from build123d import *

# Parameters (mm, degrees)
SKETCH1_R               = 20
BOSS_EXTRUDE1_DEPTH     = 142.5
SKETCH2_R               = 24
BOSS_EXTRUDE2_DEPTH     = 15
SKETCH3_R               = 20
BOSS_EXTRUDE3_DEPTH     = 40
SKETCH5_R               = 15
BOSS_EXTRUDE4_DEPTH     = 45
CUT_EXTRUDE1_DEPTH      = 245.863737617
CUT_EXTRUDE1_DEPTH_BACK = 245.863737617
SKETCH4_R               = 11.5
SKETCH7_W               = 2
SKETCH7_H               = 1.5
SKETCH10_W              = 2.5
SKETCH10_H              = 50.5


with BuildPart() as part:
    # Sketch1 → Boss-Extrude1 (new body)
    with BuildSketch(Plane(origin=(0, 0, 0), x_dir=(1, 0, 0), z_dir=(0, 1, 0))):
        with Locations(Location((0, 0, 0), (0, 0, 270))):
            Circle(SKETCH1_R)
    extrude(amount=BOSS_EXTRUDE1_DEPTH)

    # Sketch2 → Boss-Extrude2 (add)
    with BuildSketch(Plane(origin=(0, 142.5, 0), x_dir=(1, 0, 0), z_dir=(0, 1, 0))):
        with Locations(Location((0, 0, 0), (0, 0, 270))):
            Circle(SKETCH2_R)
    extrude(amount=BOSS_EXTRUDE2_DEPTH)

    # Sketch3 → Boss-Extrude3 (add)
    with BuildSketch(Plane(origin=(0, 157.5, 0), x_dir=(1, 0, 0), z_dir=(0, 1, 0))):
        with Locations(Location((-0.463755605, 0, 0), (0, 0, 270))):
            Circle(SKETCH3_R)
    extrude(amount=BOSS_EXTRUDE3_DEPTH)

    # Sketch5 → Boss-Extrude4 (add)
    with BuildSketch(Plane.XZ):
        with Locations(Location((0, 0, 0), (0, 0, 90))):
            Circle(SKETCH5_R)
    extrude(amount=BOSS_EXTRUDE4_DEPTH)

    # Sketch4 → Cut-Extrude1 (cut, two sides: drawn at the far end of the back side and taken through both)
    with BuildSketch(Plane(origin=(0, 197.5, 0), x_dir=(1, 0, 0), z_dir=(0, 1, 0)).offset(-CUT_EXTRUDE1_DEPTH_BACK)):
        with Locations(Location((0, 0, 0), (0, 0, 270))):
            Circle(SKETCH4_R)
    extrude(amount=CUT_EXTRUDE1_DEPTH + CUT_EXTRUDE1_DEPTH_BACK, mode=Mode.SUBTRACT)

    # Sketch7 → Cut-Revolve1 (revolve, cut)
    with BuildSketch(Plane(origin=(0, 0, 0), x_dir=(0, 0, -1), z_dir=(1, 0, 0)), mode=Mode.PRIVATE) as cut_revolve1_sk:
        with Locations((14, -40.75)):
            Rectangle(SKETCH7_W, SKETCH7_H)
    revolve(cut_revolve1_sk.sketch.rotate(Axis((0, -40.130931017, 0), (0, 1, 0)), 180), axis=Axis((0, -40.130931017, 0), (0, 1, 0)), mode=Mode.SUBTRACT)

    # Sketch10 → Cut-Revolve2 (revolve, cut)
    with BuildSketch(Plane.XY, mode=Mode.PRIVATE) as cut_revolve2_sk:
        with Locations((-18.75, 25.25)):
            Rectangle(SKETCH10_W, SKETCH10_H)
    revolve(cut_revolve2_sk.sketch.rotate(Axis((0, -22.168396133, 0), (0, 1, 0)), 270), axis=Axis((0, -22.168396133, 0), (0, 1, 0)), mode=Mode.SUBTRACT)


solid = part.part
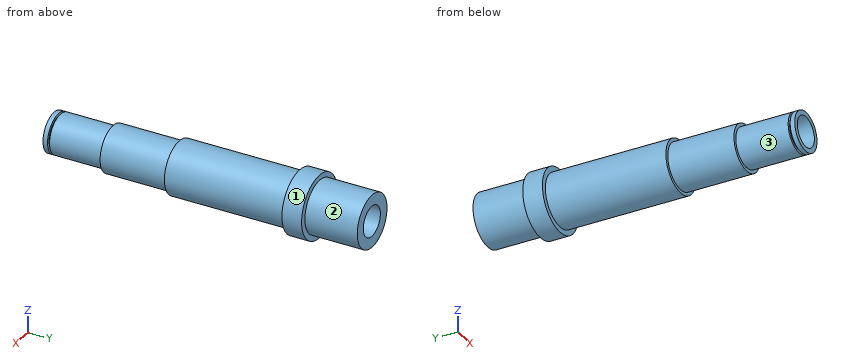
For this review, take the finished solid that the model builds, in its own axes (mm). Face numbers are marked on the shaded views. A direction names the side the tool comes from. Coordinates: 2 decimals unless noted, no trailing zeros. Loops run counter-clockwise (first coordinate to the right, second up) from the corner with the lowest first, then second, coordinate; pieces in that order, holes last. Notation, with made-up numbers: (-19, 76) - (29, 76) arc R26 ccw to (29, 92) - close; hole circle Ø5 at (5, 29). An arc over 180 degrees is marked (long way). Return JSON: item names as keys, results as strings.
Item 1: For the marked faces 1, 2 and 3, list the 3-axis set-ups (+Z, -Z, +X, -X, +Y, -Y) from which the entire face can be reached by the end or side of a thin tool; tool diameter is ignored.
Determined:
{"face 1": "+Y, -Y", "face 2": "+Y", "face 3": "-Y"}
Item 2: Take a section at C-C (y = 102). Give the boundary of the cut face in (x, z), then the cut area to 3 significant figures.
Determined:
{"outline": "circle Ø40 at (0, 0); hole circle Ø23 at (0, 0)", "area": "841 mm2"}
Item 3: For line 1 (X direction, y = 123, z = 0); line 2 (X direction, y = 32, z = 0); line 3 (Y direction, x = 17, z = 9), list the stretches that pass through material, from the lowest coordinate up.
Determined:
{"line 1": "x = -20 to -11.5, 11.5 to 20", "line 2": "x = -17.5 to -11.5, 11.5 to 17.5", "line 3": "y = 50.5 to 197.5"}
Item 4: Insertion check: pin 1 (24 mm diameter, centred on x = 5.5, z = -2, fed in from -Y); pin 2 (2 mm diameter, centred on y = 29, z = 2, fed in from +X); pin 3 (20.5 mm diameter, centred on x = 0, z = 0, fed in from -Y); pin 4 (10 mm diameter, centred on x = 17, y = -18.5, fed in from +Z). Each pin has a flat end and moves straight along its axis. Give the tip position at first contact, or say it passes through.
Determined:
{"pin 1": "stops at y = -45", "pin 2": "stops at x = 17.47", "pin 3": "passes through", "pin 4": "stops at z = 9"}
